Drawing for the job (mm, zero at the part's lowest x, y, z). Coordinates: 2 decimals unless noted, no trailing zeros. Loops run counter-clockwise (first coordinate to the right, second up) from the corner with the lowest first, then second, coordinate; pieces in that order, holes last. Notation, with made-up numbers: (28, 41) -> (79, 41) arc R7 ccw to (79, 49) -> close; hole circle Ø3 at (7.5, 16.5). An arc over 180 degrees is marked (long way). Write each question's results on one line, items separated by ' | '.
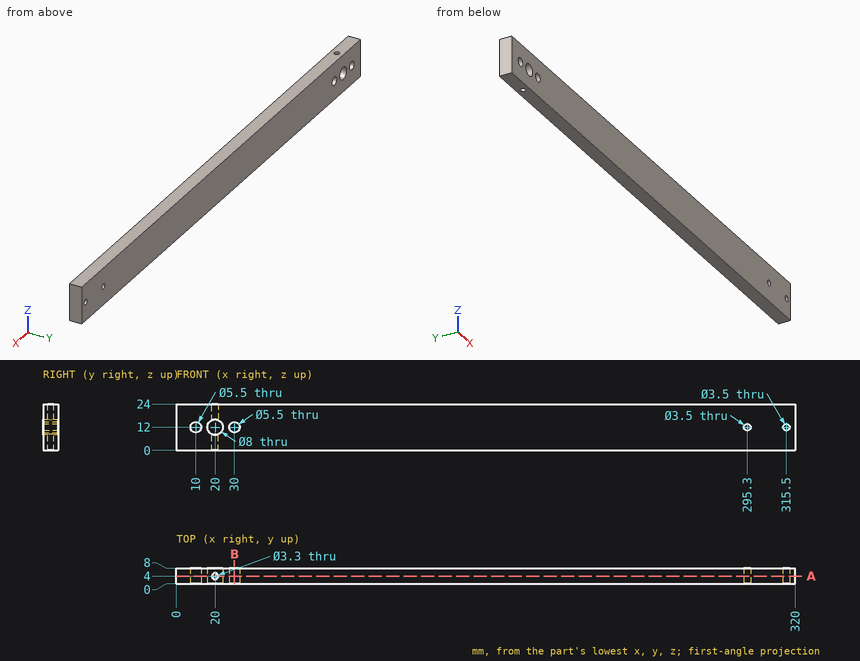
1) Drill centre lines: L1, parallel to X at y = 4, z = 12; L2, parallel to X at y = 3.75, z = 18.5; L3, parallel to Y at x = 20, z = 22.5. Where is each one in solid material? Low to high. Write a range as from..to.
Outcome:
L1: x = 0..7.25, 12.75..16, 24..27.25, 32.75..293.55, 297.05..313.75, 317.25..320 | L2: x = 0..18.37, 21.63..320 | L3: y = 0..2.35, 5.65..8
2) Slice it at B-B (x = 30). Write the cut outline in (y, z), then the cut area to 3 significant figures.
Outcome:
outline: (0, 0) -> (8, 0) -> (8, 9.25) -> (0, 9.25) -> close; (0, 14.75) -> (8, 14.75) -> (8, 24) -> (0, 24) -> close | area: 148 mm^2
3) Slice it at A-A (y = 4). Write the cut outline in (x, z), then the cut area to 3 significant figures.
Outcome:
outline: (0, 0) -> (18.35, 0) -> (18.35, 8.36) arc R4 cw to (18.35, 15.64) -> (18.35, 24) -> (0, 24) -> close; (21.65, 0) -> (320, 0) -> (320, 24) -> (21.65, 24) -> (21.65, 15.64) arc R4 cw to (21.65, 8.36) -> close; hole circle Ø5.5 at (10, 12); hole circle Ø5.5 at (30, 12); hole circle Ø3.5 at (295.3, 12); hole circle Ø3.5 at (315.5, 12) | area: 7,510 mm^2
